Part model, mm, in its own coordinate system. A direction names the side the tool comes from. Coordinates: 2 decimals unless noted, no trailing zeros. Order: outer loops, then holes, each group sorted by start corner. A loop starts at its lowest first (then second) coordinate and runs counter-clockwise, first axis right, second up. Notation, with made-up numbers: (69.5, 83) - (117.5, 83) arc R14 ccw to (117.5, 109) - close; hole circle Ø2 at (50.5, -2). An arc over 180 degrees is marked (long way). Use a Markdown table: item, result. Add a question column.
1) Tool access for faces 1 (the face through (42, 2, -11)), 2 (the face through (114.36, 2, -40)), 3 (the face through (99, 2, -69.57)), 4 (the face through (88.06, 2, -8)), 5 (the face through (1.5, 2.2, -73.3)): list every direction of +Z, -Z, +X, -X, +Y, -Y with a clear straight run to the whole face (end or side of a thin tool).
2) Two-plate mould, pull along Z, no slides. Class faces 6 (the face through (56, 4.55, -38)), 7 (the face through (86.56, 2.24, -1.43)), 8 (the face through (31.2, 2.2, -27.9)): +Z half, -Z half, draft (parallel to the pull), parting line (faces both ways), or undercut.
3) Saw through at A-A on x = 33.35. List the corners of the cut face in (y, z).
4) Saw through at C-C on x = 63.15. List the corners of the cut face in (y, z).
5) Drop flat-ended pins along their axis: P1, Ø1.7, axis at x = 63.15, z = -4.8, coming from the -Y side; P2, Ø1.4, axis at x = 102.5, y = 3, coming from the +Z side. Give the stop position or say it passes through.
6) Saw through at D-D on z = -27.83. List the corners of the cut face in (x, y), then the cut area to 3 significant figures.
7) Wall check: L1, parallel to X at y = 1.95, z = -60; L2, parallel to Z at x = 80.65, y = 2; L3, parallel to Z at x = 94.47, y = 1.4. Give the ranges that are in metal, low to high. Write a range as [from, to].
8) Saw through at B-B on z = -39.69. List the corners of the cut face in (x, y), then the cut area to 3 significant figures.
```python
from build123d import *

# Parameters (mm, degrees)
SKETCH1_R           = 2.15
SKETCH1_R_2         = 6.15
SKETCH1_R_3         = 1.75
SKETCH1_R_4         = 1.4
SKETCH1_W           = 7.3
SKETCH1_H           = 3.2
BOSS_EXTRUDE1_DEPTH = 4.55


with BuildPart() as part:
    # Sketch1 → Boss-Extrude1 (new body)
    with BuildSketch(Plane(origin=(0, 0, 0), x_dir=(1, 0, 0), z_dir=(0, 1, 0))):
        with BuildLine():
            Line((5, 0), (83.06, 0))
            ThreePointArc((83.06, 0), (86.595533906, 1.464466094), (88.06, 5))
            Line((88.06, 5), (88.06, 10.2))
            Line((88.06, 10.2), (109.36, 10.2))
            ThreePointArc((109.36, 10.2), (112.895533906, 11.664466094), (114.36, 15.2))
            Line((114.36, 15.2), (114.36, 64.57))
            ThreePointArc((114.36, 64.57), (112.895533906, 68.105533906), (109.36, 69.57))
            Line((109.36, 69.57), (88.06, 69.57))
            Line((88.06, 69.57), (88.06, 69.73))
            ThreePointArc((88.06, 69.73), (86.595533906, 73.265533906), (83.06, 74.73))
            Line((83.06, 74.73), (5, 74.73))
            ThreePointArc((5, 74.73), (1.464466094, 73.265533906), (0, 69.73))
            Line((0, 69.73), (0, 5))
            ThreePointArc((0, 5), (1.464466094, 1.464466094), (5, 0))
        make_face()
        with Locations((5.15, 59.83)):
            Circle(SKETCH1_R, mode=Mode.SUBTRACT)
        with Locations((33.35, 59.83)):
            Circle(SKETCH1_R, mode=Mode.SUBTRACT)
        with Locations((52.45, 59.83)):
            Circle(SKETCH1_R, mode=Mode.SUBTRACT)
        with Locations((80.65, 59.83)):
            Circle(SKETCH1_R, mode=Mode.SUBTRACT)
        with Locations((5.15, 27.83)):
            Circle(SKETCH1_R, mode=Mode.SUBTRACT)
        with Locations((33.35, 27.83)):
            Circle(SKETCH1_R, mode=Mode.SUBTRACT)
        with Locations((52.45, 27.83)):
            Circle(SKETCH1_R, mode=Mode.SUBTRACT)
        with Locations((80.65, 27.83)):
            Circle(SKETCH1_R, mode=Mode.SUBTRACT)
        with Locations((94.47, 39.69)):
            Circle(SKETCH1_R_2, mode=Mode.SUBTRACT)
        with Locations((94.45, 65.33)):
            Circle(SKETCH1_R_3, mode=Mode.SUBTRACT)
        with Locations((94.45, 15.69)):
            Circle(SKETCH1_R_3, mode=Mode.SUBTRACT)
        with Locations((63.15, 4.8)):
            Circle(SKETCH1_R_4, mode=Mode.SUBTRACT)
        with Locations((72.95, 4.8)):
            Circle(SKETCH1_R_4, mode=Mode.SUBTRACT)
        with Locations((42.45, 70.13)):
            Rectangle(SKETCH1_W, SKETCH1_H, mode=Mode.SUBTRACT)
        with Locations((42.45, 9.4)):
            Rectangle(SKETCH1_W, SKETCH1_H, mode=Mode.SUBTRACT)
    extrude(amount=BOSS_EXTRUDE1_DEPTH)


solid = part.part
```
Results are:
| question | item | result |
|---|---|---|
| 1 | face 1 | +Y, -Y |
| 1 | face 2 | +Z, -Z, +X, +Y, -Y |
| 1 | face 3 | -Z, +X, +Y, -Y |
| 1 | face 4 | +Z, +X, +Y, -Y |
| 1 | face 5 | -Z, -X, +Y, -Y |
| 2 | face 6 | draft |
| 2 | face 7 | +Z half |
| 2 | face 8 | undercut |
| 3 | outline | (0, -74.73) - (4.55, -74.73) - (4.55, -61.98) - (0, -61.98) - close; (0, -57.68) - (4.55, -57.68) - (4.55, -29.98) - (0, -29.98) - close; (0, -25.68) - (4.55, -25.68) - (4.55, 0) - (0, 0) - close |
| 4 | outline | (0, -74.73) - (4.55, -74.73) - (4.55, -6.2) - (0, -6.2) - close; (0, -3.4) - (4.55, -3.4) - (4.55, 0) - (0, 0) - close |
| 5 | P1 | through |
| 5 | P2 | z = -10.2 |
| 6 | outline | (0, 0) - (3, 0) - (3, 4.55) - (0, 4.55) - close; (7.3, 0) - (31.2, 0) - (31.2, 4.55) - (7.3, 4.55) - close; (35.5, 0) - (50.3, 0) - (50.3, 4.55) - (35.5, 4.55) - close; (54.6, 0) - (78.5, 0) - (78.5, 4.55) - (54.6, 4.55) - close; (82.8, 0) - (114.36, 0) - (114.36, 4.55) - (82.8, 4.55) - close |
| 6 | area | 442 mm2 |
| 7 | L1 | [0, 3.01], [7.29, 31.21], [35.49, 50.31], [54.59, 78.51], [82.79, 114.36] |
| 7 | L2 | [-74.73, -61.98], [-57.68, -29.98], [-25.68, 0] |
| 7 | L3 | [-69.57, -67.08], [-63.58, -45.84], [-33.54, -17.44], [-13.94, -10.2] |
| 8 | outline | (0, 0) - (88.32, 0) - (88.32, 4.55) - (0, 4.55) - close; (100.62, 0) - (114.36, 0) - (114.36, 4.55) - (100.62, 4.55) - close |
| 8 | area | 464 mm2 |
